Autodesk Fusion 360 part; units mm, degrees
sketch "Sketch1" plane through (0, 0, 0) normal (0, 0, 1) x (1, 0, 0)
  circle A0 centre (0, 0) radius 10
  circle A1 centre (0, 0) radius 12.5
  circle A2 centre (0, 0) radius 15
  dimension "d1" = 20
  dimension "d2" = 25
  dimension "d3" = 30
extrude "Extrude1" add sketch "Sketch1" along normal blind 25 contours A1
extrude "Extrude2" add sketch "Sketch1" along normal blind 5 contours A2
extrude "Extrude3" add sketch "Sketch1" along normal blind 5 contours A0
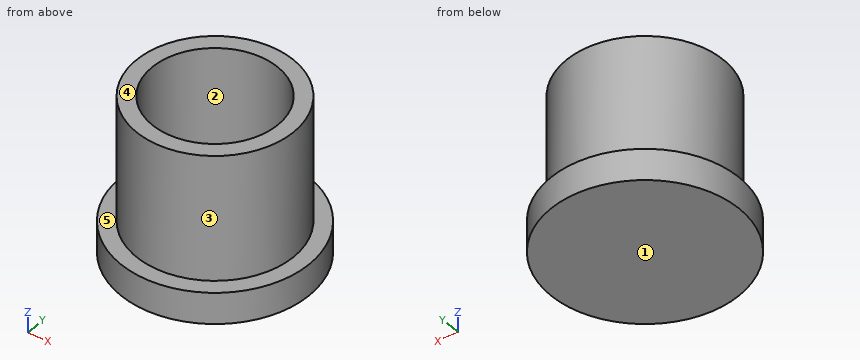
Input: part model. Units: mm. Frame: model coordinates. Face numbers are marked on the shaded views. A direction names the side the tool comes from. Round coordinates to 2 decimals unless told otherwise and drop trailing zeros. Loops run counter-clockwise (first coordinate to the right, second up) from the corner with the lowest first, then second, coordinate; pieces in that order, holes last. Notation, with made-up numbers: M 81,-37.75 L 137,-37.75 A24 ccw 137,-25.75 Z; hole C 40,-13 d3. An arc over 180 degrees is marked long. Answer as CSV lines item,"result". Start each with the question number.
(1) Section A-A, the plane x = 0. Output: boundary loops of the cut face in (y, z).
(2) Reachability of the marked faces 4 and 5 from +Z, -Z, +X, -X, +Y, -Y: full face, straight path, thin tool, end or side. Return the list, or none.
(3) Section C-C, the plane z = 20. Output: boundary loops of the cut face in (x, y), plus the area to 3 significant figures.
(4) Draft query along X for the marked faces 1, 2 and 3. Return one class per face: released by +X, released by -X, zero draft, split by the parting line, or undercut.
(5) First-contact query: pin 1 (12 mm diameter, centred on y = 4.5, z = 13, fed in from -X); pin 2 (6 mm diameter, centred on x = -5.5, y = 11, fed in from -Z); pin 3 (2 mm diameter, centred on x = -1.5, y = -5, fed in from +Z); pin 4 (1 mm diameter, centred on y = 5.5, z = 20.5, fed in from -X). Flat tips, straight axial feed; report the tip coordinate or a pass-through.
(6) Line query: line 1 (Y direction, x = 0, z = 18.75); line 2 (X direction, y = -6, z = 6); line 3 (X direction, y = -0.5, z = 7). Output: solid intervals per line, ascending. Write a range as [from, to].
(7) Section D-D, the plane z = 2. Output: boundary loops of the cut face in (x, y), plus the area to 3 significant figures.
Values found:
1,outline,"M -15,0 L 15,0 L 15,5 L 12.5,5 L 12.5,25 L 10,25 L 10,5 L -10,5 L -10,25 L -12.5,25 L -12.5,5 L -15,5 Z"
2,face 4,"+Z, +X, -X, +Y, -Y"
2,face 5,"+Z"
3,outline,"C 0,0 d25; hole C 0,0 d20"
3,area,"177 mm²"
4,face 1,"zero draft"
4,face 2,"undercut"
4,face 3,"split by the parting line"
5,pin 1,"stops at x = -12.5"
5,pin 2,"stops at z = 0"
5,pin 3,"stops at z = 5"
5,pin 4,"stops at x = -11.46"
6,line 1,"y = [-12.5, -10], [10, 12.5]"
6,line 2,"x = [-10.97, -8], [8, 10.97]"
6,line 3,"x = [-12.49, -9.99], [9.99, 12.49]"
7,outline,"C 0,0 d30"
7,area,"707 mm²"
